For this review, use the dimensioned drawing (mm, ordinates from the lowest corner) and the shaded views. Round coordinates to 2 decimals unless told otherwise and drop trailing zeros. Write each loop counter-clockwise with the first axis right and the second up, starting at its lowest first coordinate (ties: lowest second). Pieces come first, ordered by that corner, then holes. Notation, with made-up numbers: (83, -10.5) -> (103, -10.5) arc R23 ccw to (103, 13.5) -> close; hole circle Ø10 at (30, 9). An arc over 180 degrees is marked (long way). Write each question's results on one line, items separated by ' | '. Start each with the question number.
Item 1: Clearance check with flat-ended pins moving along their axes: pin 1 (3 mm diameter, centred on x = 84.5, y = 3, fed in from -Z); pin 2 (2 mm diameter, centred on y = 0.5, z = 16.5, fed in from -X); pin 3 (4.5 mm diameter, centred on x = 109.79, z = 109.79, fed in from -Y). State where each tip first meets the part, or that it passes through.
Item 2: Add section D-D (z = 17.5). State the section outline as (x, y) points.
Item 3: Add section A-A (y = 1.3). State the section outline as (x, z) points, plus the area to 3 significant figures.
Item 4: Add section B-B (x = 110). State the section outline as (y, z) points, plus the area to 4 significant figures.
Item 5: To check wall thickness, follow line 1 along X through (y, z) = (3.75, 109.79); line 2 along X through (y, z) = (2.5, 75). State the ranges of each line that lie inside material, in increasing order.
Item 6: Add section C-C (z = 109.79). State the section outline as (x, y) points, plus the area to 3 significant figures.
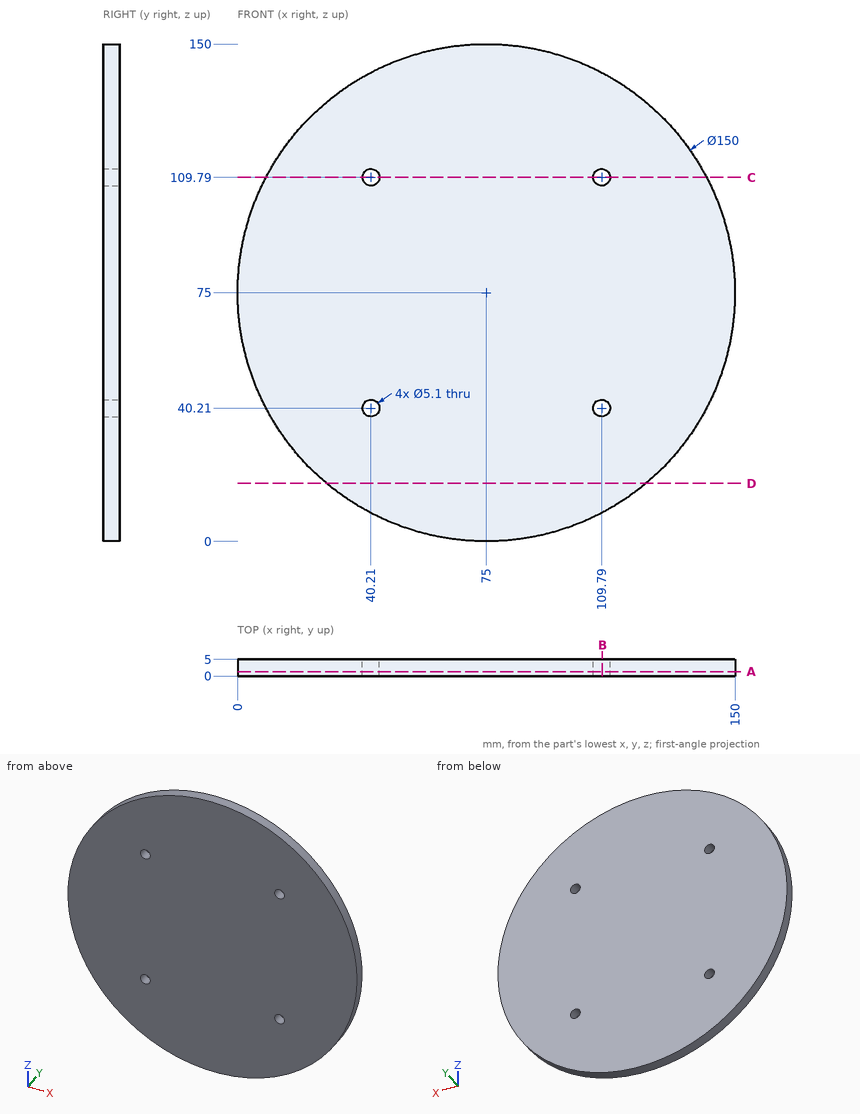
Responses:
1) pin 1: stops at z = 0.43 | pin 2: stops at x = 26.85 | pin 3: passes through
2) outline: (26.85, 0) -> (123.15, 0) -> (123.15, 5) -> (26.85, 5) -> close
3) outline: circle Ø150 at (75, 75); hole circle Ø5.1 at (40.21, 40.21); hole circle Ø5.1 at (40.21, 109.79); hole circle Ø5.1 at (109.79, 40.21); hole circle Ø5.1 at (109.79, 109.79) | area: 17,600 mm^2
4) outline: (0, 8.67) -> (5, 8.67) -> (5, 37.67) -> (0, 37.67) -> close; (0, 42.75) -> (5, 42.75) -> (5, 107.25) -> (0, 107.25) -> close; (0, 112.33) -> (5, 112.33) -> (5, 141.33) -> (0, 141.33) -> close | area: 612.5 mm^2
5) line 1: x = 8.56 to 37.66, 42.76 to 107.24, 112.34 to 141.44 | line 2: x = 0 to 150
6) outline: (8.56, 0) -> (37.66, 0) -> (37.66, 5) -> (8.56, 5) -> close; (42.76, 0) -> (107.24, 0) -> (107.24, 5) -> (42.76, 5) -> close; (112.34, 0) -> (141.44, 0) -> (141.44, 5) -> (112.34, 5) -> close | area: 613 mm^2
